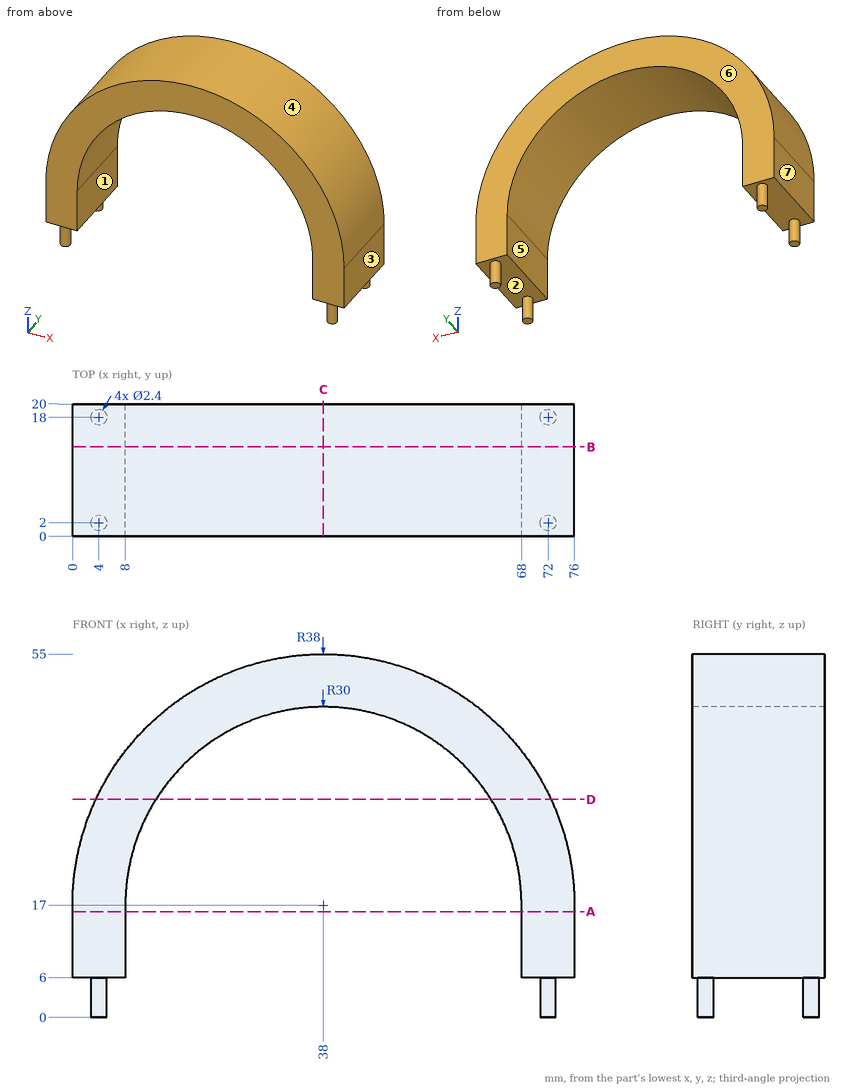
Verification items for this drawing (mm, ordinates from the low corner). A direction names the side the tool comes from. Round coordinates to 2 decimals unless told otherwise and drop trailing zeros. Loops run counter-clockwise (first coordinate to the right, second up) from the corner with the lowest first, then second, coordinate; pieces in that order, holes last. Notation, with made-up numbers: (21, 73) -> (35, 73) arc R6 cw to (35, 81) -> close; hole circle Ø8 at (53.5, -14). An arc over 180 degrees is marked (long way). Write item = value, one per line. Start each with the question number.
1) Sectioned sample at B-B, the plane y = 13.5. Record the cut outline in (x, z).
2) Sectioned sample at A-A, the plane z = 16. Record the cut outline in (x, y).
3) Sectioned sample at D-D, the plane z = 33. Record the cut outline in (x, y), plus the area to 3 significant figures.
4) Gauge pin test, flat ends, axial feed: pin 1 Ø2.5 at (x, y) = (3, 11.5) entering from -Z; pin 2 Ø1 at (x, y) = (11, 13) entering from -Z; pin 3 Ø9 at (x, y) = (71, 14) entering from -Z; pin 4 Ø6 at (x, y) = (52.5, 4) entering from -Z. Record the tip position at first contact, or that the pin passes through.
5) Sectioned sample at C-C, the plane x = 38. Record the cut outline in (y, z).
6) Set-up check for the marked faces 1, 2 and 3: record each of +Z, -Z, +X, -X, +Y, -Y from which the full face is reachable in a straight line by a thin tool's end or side.
7) Release check for a two-part mould opening along X. For the marked faces 4, 5, 6 and 7 record: released by +X, released by -X, zero draft, split by the parting line, or undercut.
8) Thickness scan on probe 1 along X at (y, z) = (13.5, 18); probe 2 along X at (y, z) = (12, 34); probe 3 along X at (y, z) = (1, 51). Record the ranges inside material, lowest first.
Results are:
q1.outline = (0, 6) -> (8, 6) -> (8, 17) arc R30 cw to (68, 17) -> (68, 6) -> (76, 6) -> (76, 17) arc R38 ccw to (0, 17) -> close
q2.outline = (0, 0) -> (8, 0) -> (8, 20) -> (0, 20) -> close; (68, 0) -> (76, 0) -> (76, 20) -> (68, 20) -> close
q3.outline = (3.53, 0) -> (12.62, 0) -> (12.62, 20) -> (3.53, 20) -> close; (63.38, 0) -> (72.47, 0) -> (72.47, 20) -> (63.38, 20) -> close
q3.area = 364 mm^2
q4.pin_1 = 6
q4.pin_2 = 28.99
q4.pin_3 = 0
q4.pin_4 = 41.37
q5.outline = (0, 47) -> (20, 47) -> (20, 55) -> (0, 55) -> close
q6.face_1 = -Z, +Y, -Y
q6.face_2 = -Z
q6.face_3 = +Z, -Z, +X, +Y, -Y
q7.face_4 = split by the parting line
q7.face_5 = undercut
q7.face_6 = zero draft
q7.face_7 = released by -X
q8.probe_1 = 0.01 to 8.02, 67.98 to 75.99
q8.probe_2 = 4.01 to 13.28, 62.72 to 71.99
q8.probe_3 = 21.03 to 54.97
